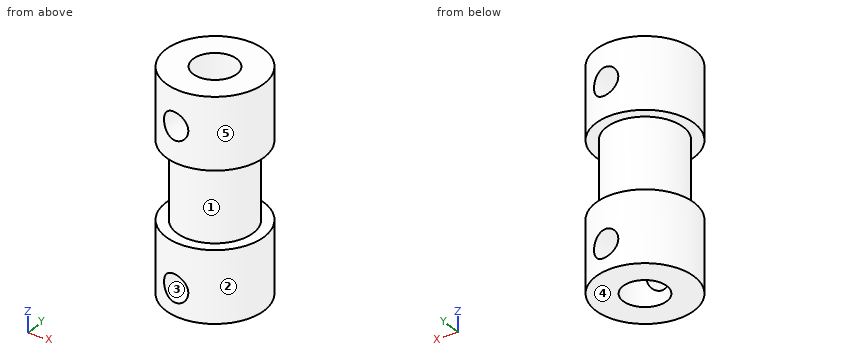
from build123d import *

# Parameters (mm, degrees)
F_4_0MM_DOWEL_HOLE1_D           = 4
M3X0_5_TAPPED_HOLE1_D           = 2.5
M3X0_5_TAPPED_HOLE1_ON_FACE_2_D = 2.5


with BuildPart() as part:
    # Sketch1 → Revolve1 (revolve)
    with BuildSketch(Plane(origin=(0, 0, 0), x_dir=(1, 0, 0), z_dir=(0, 1, 0))):
        Polygon((4.5, 10), (0, 10), (0, -10), (4.5, -10), (4.5, -3.5), (3.5, -3.5), (3.5, 3.5), (4.5, 3.5), align=None)
    revolve(axis=Axis((0, 0, -10), (0, 0, 1)))

    # Ø4.0mm Dowel Hole1 (through all)
    with Locations(Plane.XY.offset(10)):
        with Locations((0, 0)):
            Hole(F_4_0MM_DOWEL_HOLE1_D / 2)

    # M3x0.5 Tapped Hole1 (through all)
    with Locations(Plane(origin=(0.688844658, 4.446964474, 6.712810899), x_dir=(0.988214328, -0.153076591, 0), z_dir=(0.153076591, 0.988214328, 0))):
        with Locations((0, 0)):
            Hole(M3X0_5_TAPPED_HOLE1_D / 2)

    # M3x0.5 Tapped Hole1 on face 2 (through all)
    with Locations(Plane(origin=(0.688844658, 4.446964474, -7.56241821), x_dir=(0.988214258, -0.15307704, 0), z_dir=(0.15307704, 0.988214258, 0))):
        with Locations((0, 0)):
            Hole(M3X0_5_TAPPED_HOLE1_ON_FACE_2_D / 2)


solid = part.part
The model under review builds one solid part; all positions refer to its coordinate system, in mm. Face numbers are marked on the shaded views. A direction names the side the tool comes from. Coordinates: 2 decimals unless noted, no trailing zeros. Order: outer loops, then holes, each group sorted by start corner. A loop starts at its lowest first (then second) coordinate and runs counter-clockwise, first axis right, second up. Notation, with made-up numbers: (28.5, -26.75) -> (52.5, -26.75) arc R22 cw to (52.5, -9.75) -> close; hole circle Ø1 at (-30.5, 40). An arc over 180 degrees is marked (long way). Answer in a Markdown table with one row per item.
(1) Wall thickness on line 1 along Z through (x, y) = (0.5, 4); line 2 along Y through (x, z) = (0, 2.5); line 3 along Y through (x, z) = (0, -4.75): over which ranges is each line inside the solid? List them lowest first.
Answers:
| item | result |
|---|---|
| line 1 | -10 to -8.81, -6.32 to -3.5, 3.5 to 5.47, 7.96 to 10 |
| line 2 | -3.5 to -2, 2 to 3.5 |
| line 3 | -4.5 to -2, 2 to 4.5 |
(2) Consider section B-B (z = 6). Write out the cut boundary in (x, y), plus the area to 3 significant figures.
Answers:
| item | result |
|---|---|
| outline | (-1.69, -4.17) -> (-1.28, -1.54) arc R2 cw to (-0.75, 1.85) -> (-0.34, 4.49) arc R4.5 ccw to start; (0.34, -4.49) arc R4.5 ccw to (1.69, 4.17) -> (1.28, 1.54) arc R2 cw to (0.75, -1.85) -> close |
| area | 40.6 mm² |
(3) Machinability: for the marked faces 1 and 2, which of the approach directions +Z, -Z, +X, -X, +Y, -Y give a long, thin tool a straight path to every point of the face, cutting with its end or side? Answer none if there is none.
Answers:
| item | result |
|---|---|
| face 1 | none |
| face 2 | +Z, -Z |
(4) Consider section A-A (y = 0). Write out the cut boundary in (x, z), plus the area to 3 significant figures.
Answers:
| item | result |
|---|---|
| outline | (-4.5, -10) -> (-2, -10) -> (-2, 10) -> (-4.5, 10) -> (-4.5, 3.5) -> (-3.5, 3.5) -> (-3.5, -3.5) -> (-4.5, -3.5) -> close; (2, -10) -> (4.5, -10) -> (4.5, -3.5) -> (3.5, -3.5) -> (3.5, 3.5) -> (4.5, 3.5) -> (4.5, 10) -> (2, 10) -> close |
| area | 86.0 mm² |
(5) The part is to be moulded in two halves that separate along X. For the marked faces 3, 4 and 5, say which applies: +X half, -X half, draft (parallel to the pull), parting line (faces both ways), or undercut.
Answers:
| item | result |
|---|---|
| face 3 | undercut |
| face 4 | draft |
| face 5 | parting line |
(6) Consider section D-D (x = 3). Write out the cut boundary in (y, z).
Answers:
| item | result |
|---|---|
| outline | (-3.35, -10) -> (3.35, -10) -> (3.35, -3.5) -> (1.8, -3.5) -> (1.8, 3.5) -> (3.35, 3.5) -> (3.35, 10) -> (-3.35, 10) -> (-3.35, 3.5) -> (-1.8, 3.5) -> (-1.8, -3.5) -> (-3.35, -3.5) -> close |
(7) Consider section C-C (z = 1.25). Write out the cut boundary in (x, y), plus the area to 3 significant figures.
Answers:
| item | result |
|---|---|
| outline | circle Ø7 at (0, 0); hole circle Ø4 at (0, 0) |
| area | 25.9 mm² |
(8) Insertion check: pin 1 (4 mm diameter, centred on x = -2.5, z = -4, fed in from -Y); pin 2 (2.5 mm diameter, centred on x = 0, y = 0, fed in from -Z); pin 3 (4 mm diameter, centred on y = -2, z = -2.5, fed in from +X); pin 4 (2 mm diameter, centred on y = -3.5, z = 2, fed in from -X). Each pin has a flat end and moves straight along its axis. Give the tip position at first contact, or say it passes through.
Answers:
| item | result |
|---|---|
| pin 1 | y = -4.47 |
| pin 2 | through |
| pin 3 | x = 4.49 |
| pin 4 | x = -2.45 |
